```python
from build123d import *

# Parameters (mm, degrees)
F0_W           = 35
F0_H           = 50.8
F1_DEPTH       = 13
F2_W           = 29
F2_H           = 7
F3_DEPTH       = 28
F4_W           = 15
F4_H           = 7
F5_DEPTH       = 35.001
F7_DEPTH       = 13.001
F9_D           = 3.7973
F9_CSINK_D     = 7.7978
F9_CSINK_ANGLE = 82


with BuildPart() as f1:
    # F0 (on Top) → F1 (new body)
    with BuildSketch(Plane.XY):
        Rectangle(F0_W, F0_H)
    extrude(amount=F1_DEPTH)

    # F2 (on face) → F3 (cut)
    with BuildSketch(Plane(origin=(0, 25.4, 0), x_dir=(-1, 0, 0), z_dir=(0, 1, 0))):
        with Locations((0, 6.5)):
            Rectangle(F2_W, F2_H)
    extrude(amount=-F3_DEPTH, mode=Mode.SUBTRACT)

    # F4 (on face) → F5 (cut, through all)
    with BuildSketch(Plane.YZ.offset(17.5)):
        with Locations((4.9, 6.5)):
            Rectangle(F4_W, F4_H)
    extrude(amount=-F5_DEPTH, mode=Mode.SUBTRACT)

    # F6 (on face) → F7 (cut, through all)
    with BuildSketch(Plane.XY.offset(13)):
        Polygon((-17.5, -25.4), (-5, -25.4), (-5, -2.6), (-10.5, 12.4), (-17.5, 12.4), (-17.5, -2.6), align=None)
        Polygon((17.5, -2.6), (17.5, 12.4), (10.5, 12.4), (5, -2.6), (5, -25.4), (17.5, -25.4), align=None)
    extrude(amount=-F7_DEPTH, mode=Mode.SUBTRACT)

    # F9 (through all)
    with Locations(Plane.XY.offset(13)):
        with Locations((0, -8.6), (0, -19.4)):
            CounterSinkHole(F9_D / 2, F9_CSINK_D / 2, counter_sink_angle=F9_CSINK_ANGLE)


solid = f1.part
```
Model file for the job. Use its own axes, mm. A direction names the side the tool comes from. Coordinates: 2 decimals unless noted, no trailing zeros. Loops run counter-clockwise (first coordinate to the right, second up) from the corner with the lowest first, then second, coordinate; pieces in that order, holes last. Notation, with made-up numbers: (84, -8.75) - (123, -8.75) arc R21 cw to (123, 2.25) - close; hole circle Ø5 at (-22, 37.25). An arc over 180 degrees is marked (long way). Answer as a JSON object with one key per item and string values. Group by question number.
(1) Two-plate mould, pull along Z, no slides. Class faces 1 (the face through (-17.5, 19, 6)), 2 (the face through (0, -2.6, 6)), 3 (the face through (0, 6, 0)): released by +Z, released by -Z, zero draft, split by the parting line, or undercut.
(2) Cut at C-C (x = 0). Give the cut face in (y, z), then the cut area to 3 significant figures.
(3) Flat gauge pins, fed straight in: pin 1 (3 mm diameter, centred on y = -10.5, z = 3, fed in from +X); pin 2 (5.5 mm diameter, centred on x = -15.5, z = 7.5, fed in from -Y); pin 3 (4 mm diameter, centred on x = -10.5, y = 7.5, fed in from -Z); pin 4 (6 mm diameter, centred on x = 0, y = -19.4, fed in from +Z). Where does each tip first touch, or does it go through?
(4) Cut at B-B (y = -19.4). Give the cut face in (x, z), then the cut area to 3 significant figures.
(5) Tool access for faces 4 (the face through (-14.5, 19, 6)), 5 (the face through (15, 12.4, 7)), 6 (the face through (-15, 12.4, 7)), 7 (the face through (0, 14, 10)): list every direction of +Z, -Z, +X, -X, +Y, -Y with a clear straight run to the whole face (end or side of a thin tool).
(6) Probe line 1 along Y through (x, z) = (0, 9); line 2 along X through (y, z) = (-19.4, 5); line 3 along X through (y, z) = (23.5, 3.25). List the from-to ranges inside material, lowest first.
(7) Cut at A-A (z = 6). Give the cut face in (x, y).
(8) Cut at D-D (x = 11.5). Give the cut face in (y, z).
Geometry says:
{
 "1": {"face 1": "zero draft", "face 2": "undercut", "face 3": "released by -Z"},
 "2": {"outline": "(-25.4, 0) - (-21.3, 0) - (-21.3, 10.7) - (-23.3, 13) - (-25.4, 13) - close; (-17.5, 0) - (-10.5, 0) - (-10.5, 10.7) - (-12.5, 13) - (-15.5, 13) - (-17.5, 10.7) - close; (-6.7, 0) - (25.4, 0) - (25.4, 3) - (-2.6, 3) - (-2.6, 10) - (25.4, 10) - (25.4, 13) - (-4.7, 13) - (-6.7, 10.7) - close", "area": "356 mm^2"},
 "3": {"pin 1": "stops at x = 5", "pin 2": "stops at y = 12.4", "pin 3": "stops at z = 0", "pin 4": "stops at z = 11.97"},
 "4": {"outline": "(-5, 0) - (-1.9, 0) - (-1.9, 10.7) - (-3.9, 13) - (-5, 13) - close; (1.9, 0) - (5, 0) - (5, 13) - (3.9, 13) - (1.9, 10.7) - close", "area": "76.0 mm^2"},
 "5": {"face 4": "+Y, -Y", "face 5": "+Z, -Z, +X, -Y", "face 6": "+Z, -Z, -X, -Y", "face 7": "+Y"},
 "6": {"line 1": "y = -25.4 to -21.3, -17.5 to -10.5, -6.7 to -2.6", "line 2": "x = -5 to -1.9, 1.9 to 5", "line 3": "x = -17.5 to -14.5, 14.5 to 17.5"},
 "7": {"outline": "(-17.5, 12.4) - (-14.5, 12.4) - (-14.5, 25.4) - (-17.5, 25.4) - close; (-5, -25.4) - (5, -25.4) - (5, -2.6) - (-5, -2.6) - close; (14.5, 12.4) - (17.5, 12.4) - (17.5, 25.4) - (14.5, 25.4) - close; hole circle Ø3.8 at (0, -19.4); hole circle Ø3.8 at (0, -8.6)"},
 "8": {"outline": "(12.4, 0) - (25.4, 0) - (25.4, 3) - (12.4, 3) - close; (12.4, 10) - (25.4, 10) - (25.4, 13) - (12.4, 13) - close"}
}
